Geometry: final body of the model. Coordinates: model frame, mm. Face numbers are marked on the shaded views. Give positions to 0.01 mm unless a question says otherwise; leave off trailing zeros. Loops run counter-clockwise (first coordinate to the right, second up) from the corner with the lowest first, then second, coordinate; pieces in that order, holes last. Notation, with made-up numbers: (-17, -39.5) -> (-1, -39.5) arc R17 cw to (-1, -20.5) -> close; hole circle Ø3 at (14.5, -21.5). An arc over 180 degrees is marked (long way). One line per item, written item: value. Start each with the question number.
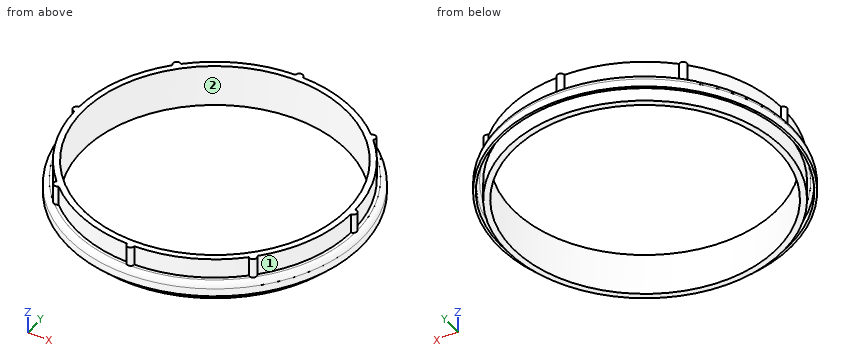
from build123d import *

# Parameters (mm, degrees)
SKETCH1_R           = 47.8155
SKETCH1_R_2         = 45.72
BOSS_EXTRUDE1_DEPTH = 7.239
SKETCH2_R           = 53.975
SKETCH2_R_2         = 47.8155
BOSS_EXTRUDE2_DEPTH = 0.41275
BOSS_EXTRUDE3_REACH = 79.693
SKETCH3_R           = 1.256285172
CIRPATTERN1_COUNT   = 8
MOVE_FACE1_BY       = 5.08


with BuildPart() as part:
    # Sketch1 → Boss-Extrude1 (new, symmetric)
    with BuildSketch(Plane.XY):
        Circle(SKETCH1_R)
        Circle(SKETCH1_R_2, mode=Mode.SUBTRACT)
    extrude(amount=BOSS_EXTRUDE1_DEPTH, both=True)

    # Sketch2 → Boss-Extrude2 (add, symmetric)
    with BuildSketch(Plane.XY):
        with Locations(Location((0, 0, 0), (0, 0, 180))):
            Circle(SKETCH2_R)
        Circle(SKETCH2_R_2, mode=Mode.SUBTRACT)
    extrude(amount=BOSS_EXTRUDE2_DEPTH, both=True)

    # Sketch3 → Boss-Extrude3 (add, up to next)
    with BuildSketch(Plane.XY.offset(7.239), mode=Mode.PRIVATE) as boss_extrude3_sk1:
        with Locations((0, 47.8155)):
            Circle(SKETCH3_R)
    boss_extrude3_tool1 = extrude(boss_extrude3_sk1.sketch, amount=-BOSS_EXTRUDE3_REACH, mode=Mode.PRIVATE) - part.part
    boss_extrude3 = boss_extrude3_tool1.solids().sort_by_distance((0, 47.8155, 7.239))[0]
    add(boss_extrude3)

    # CirPattern1: Boss-Extrude3 ×8 about axis
    cirpattern1_axis = Axis((0, 0, 0), (0, 0, 1))
    for i in range(1, CIRPATTERN1_COUNT):
        add(boss_extrude3.rotate(cirpattern1_axis, i * 360 / CIRPATTERN1_COUNT))

    # Move Face1: a curved face moved inward by 5.08
    add(Solid.thicken(part.faces().sort_by_distance((53.975, 0, 0))[0], -MOVE_FACE1_BY), mode=Mode.SUBTRACT)

    # Sketch4 → Revolve2 (revolve)
    with BuildSketch(Plane(origin=(0, 0, 0), x_dir=(0, 0, -1), z_dir=(1, 0, 0)), mode=Mode.PRIVATE) as revolve2_sk:
        with BuildLine():
            Line((-0.41275, 48.890682026), (0.41275, 48.890682026))
            ThreePointArc((0.41275, 48.890682026), (0.730192935, 49.657057065), (1.496567974, 49.9745))
            Line((1.496567974, 49.9745), (4.240158679, 49.9745))
            Line((4.240158679, 49.9745), (4.240158679, 50.8))
            Line((4.240158679, 50.8), (1.496567974, 50.8))
            ThreePointArc((1.496567974, 50.8), (0.146476287, 50.240773713), (-0.41275, 48.890682026))
        make_face()
    revolve(revolve2_sk.sketch.rotate(Axis((0, 0, -29.740513721), (0, 0, 1)), 90), axis=Axis((0, 0, -29.740513721), (0, 0, 1)))


solid = part.part
Item 1: Pin query (flat end, axial travel): pin 1 (0.5 mm diameter, centred on x = -35, y = -34.5, fed in from -Z); pin 2 (1 mm diameter, centred on x = -10, z = -3.5, fed in from +Y); pin 3 (0.5 mm diameter, centred on x = 34.5, y = -34.5, fed in from -Z). Return the tip coordinate at first contact, or that it passes through.
Item 2: Section A-A, the plane z = -2.75. Output: boundary loops of the cut face in (x, y), then the cut area to 3 significant figures.
Item 3: Mould query, pull axis X, two halves, no side actions, for the marked faces 1 and 2. Classes: pulls with the +X half, pulls with the -X half, needs draft (parallel to the pull), parting line crosses it, or undercut.
Item 4: Ray query, line 1 along Y through (x, z) = (-4.5, -3.25); line 2 along Y through (x, z) = (19.5, -1.25); line 3 along Y through (x, z) = (0, 1). Return the intervals inside material, ascending. Write a range as [from, to].
Geometry check:
1. pin 1: stops at z = -0.54
1. pin 2: stops at y = 49.9
1. pin 3: stops at z = -0.42
2. outline: circle Ø101.6 at (0, 0); circle Ø95.63 at (0, 0); hole circle Ø99.95 at (0, 0); hole circle Ø91.44 at (0, 0)
2. area: 877 mm2
3. face 1: pulls with the +X half
3. face 2: undercut
4. line 1: y = [-50.6, -49.77], [-47.6, -45.5], [45.5, 47.6], [49.77, 50.6]
4. line 2: y = [-46.89, -45.98], [-43.66, -41.35], [41.35, 43.66], [45.98, 46.89]
4. line 3: y = [-49.07, -45.72], [45.72, 49.07]
